Here's how the part is built. I have some questions about the finished solid (model axes, mm). Face numbers are marked on the shaded views. Give positions to 0.01 mm unless a question says otherwise; leave off trailing zeros. Loops run counter-clockwise (first coordinate to the right, second up) from the corner with the lowest first, then second, coordinate; pieces in that order, holes last. Notation, with made-up numbers: (29, 26.25) - (85, 26.25) arc R8 cw to (85, 36.25) - close; hole circle Ø6 at (-26, -29). An arc over 180 degrees is marked (long way). One line per item, written item: value. Start each with the question number.
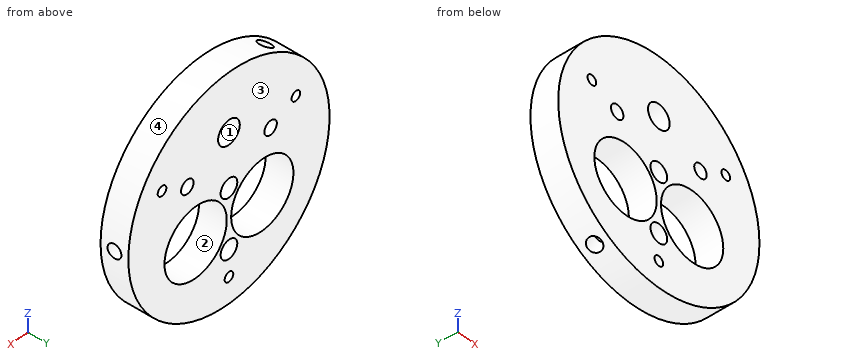
```python
from build123d import *

# Parameters (mm, degrees)
SKETCH1_R               = 38.354
BOSS_EXTRUDE1_DEPTH     = 9.525
SKETCH2_R               = 1.651
SKETCH2_R_2             = 4.1275
SKETCH2_R_3             = 11.8745
SKETCH2_R_4             = 3.175
CUT_EXTRUDE1_DEPTH      = 10.525
SKETCH4_R               = 2.3749
CUT_EXTRUDE2_DEPTH      = 6.35
CIRPATTERN1_COUNT       = 3
SKETCH5_R               = 2.38125
CUT_EXTRUDE3_DEPTH      = 1.0000001
CUT_EXTRUDE3_DEPTH_BACK = 10.5250001


with BuildPart() as part:
    # Sketch1 → Boss-Extrude1 (new body)
    with BuildSketch(Plane(origin=(0, 0, 0), x_dir=(1, 0, 0), z_dir=(0, 1, 0))):
        Circle(SKETCH1_R)
    extrude(amount=BOSS_EXTRUDE1_DEPTH)

    # Sketch2 → Cut-Extrude1 (cut, through all)
    with BuildSketch(Plane(origin=(0, 9.525, 0), x_dir=(1, 0, 0), z_dir=(0, 1, 0))):
        with Locations((0, 29.464)):
            Circle(SKETCH2_R)
        with Locations((25.516572497, -14.732)):
            Circle(SKETCH2_R)
        with Locations((-25.516572497, -14.732)):
            Circle(SKETCH2_R)
        with Locations((0, -18.415)):
            Circle(SKETCH2_R_2)
        with Locations((-12.7, 10.16)):
            Circle(SKETCH2_R_3)
        with Locations((12.7, 10.16)):
            Circle(SKETCH2_R_3)
        with Locations((0, 20.32)):
            Circle(SKETCH2_R_4)
        Circle(SKETCH2_R_4)
    extrude(amount=-CUT_EXTRUDE1_DEPTH, mode=Mode.SUBTRACT)

    # Sketch4 → Cut-Extrude2 (cut)
    with BuildSketch(Plane(origin=(-19.177, 0, -33.215538337), x_dir=(0, -1, 0), z_dir=(-0.5, 0, -0.866025404))):
        with Locations((-4.7625, 0)):
            Circle(SKETCH4_R)
    cut_extrude2 = extrude(amount=-CUT_EXTRUDE2_DEPTH, mode=Mode.SUBTRACT)

    # CirPattern1: Cut-Extrude2 ×3 about axis
    cirpattern1_axis = Axis((0, 0, 0), (0, 1, 0))
    for i in range(1, CIRPATTERN1_COUNT):
        add(cut_extrude2.rotate(cirpattern1_axis, i * 360 / CIRPATTERN1_COUNT), mode=Mode.SUBTRACT)

    # Sketch5 → Cut-Extrude3 (cut, two sides)
    with BuildSketch(Plane(origin=(0, 9.525, 0), x_dir=(1, 0, 0), z_dir=(0, 1, 0))) as cut_extrude3_sk:
        with Locations((-15.875, -10.16)):
            Circle(SKETCH5_R)
        with Locations((15.875, -10.16)):
            Circle(SKETCH5_R)
    extrude(amount=CUT_EXTRUDE3_DEPTH, mode=Mode.SUBTRACT)
    extrude(cut_extrude3_sk.sketch, amount=-CUT_EXTRUDE3_DEPTH_BACK, mode=Mode.SUBTRACT)


solid = part.part
```
(1) If we section it at D-D on z = 11.5: List the corners of the cut face in (x, y) for me (3 decimals).
(2) If we section it at B-B on x = -8: List the corners of the cut face in (y, z) for me (3 decimals), plus the area to 3 significant figures.
(3) If we section it at C-C on y = 4.5: Give the number of separate pieces and of enclosed holes in the cut face, plus the area to 3 significant figures.
(4) If we mould it in two halves opening along X, with no side actions, what happens to the marked faces 1, 2, 3 and 4? For each: pulls with the +X half, pulls with the -X half, needs draft (parallel to the pull), parting line crosses it, or undercut.
(5) Will these pins go through, and if not, where does the flat tip stop? pin 1 (10 mm diameter, centred on x = 0, z = 0, fed in from +Y) (3 decimals); pin 2 (3 mm diameter, centred on x = -1.5, y = 5, fed in from -Z); pin 3 (4 mm diameter, centred on y = 4.76, z = 0, fed in from +X); pin 4 (3 mm diameter, centred on y = 5.5, z = -28.5, fed in from +X).
(6) If we section it at A-A on z = -16: List the corners of the cut face in (x, y) for me (3 decimals), plus the area to 3 significant figures.
(7) Please list where these lines run through material, in increasing order: probe 1 along Z at (x, y) = (0, 4.75) (1 decimal); probe 2 along Z at (x, y) = (-16.5, 9.25); probe 3 along X at (y, z) = (6.5, 14). Write a range as from..to.
Found:
1. outline: (-36.589, 0) - (-17.843, 0) - (-17.843, 9.525) - (-36.589, 9.525) - close; (-13.907, 0) - (13.907, 0) - (13.907, 9.525) - (-13.907, 9.525) - close; (17.843, 0) - (36.589, 0) - (36.589, 9.525) - (17.843, 9.525) - close
2. outline: (0, -37.51) - (9.525, -37.51) - (9.525, -21.065) - (0, -21.065) - close; (0, 0.745) - (9.525, 0.745) - (9.525, 37.51) - (0, 37.51) - close
2. area: 507 mm^2
3. separate pieces: 1
3. enclosed holes: 10
3. area: 3,470 mm^2
4. face 1: undercut
4. face 2: undercut
4. face 3: needs draft
4. face 4: parting line crosses it
5. pin 1: y = 9.525
5. pin 2: z = -38.35
5. pin 3: x = 32
5. pin 4: x = 27.24
6. outline: (-34.857, 0) - (-23.039, 0) - (-23.039, 9.525) - (-34.857, 9.525) - close; (-2.361, 0) - (2.361, 0) - (2.361, 9.525) - (-2.361, 9.525) - close; (23.039, 0) - (34.857, 0) - (34.857, 9.525) - (23.039, 9.525) - close
6. area: 270 mm^2
7. probe 1: -38.4..-31.1, -27.8..-23.5, -17.1..-3.2, 3.2..14.3, 22.5..38.4
7. probe 2: -34.62..-21.41, 1.09..7.86, 12.46..34.62
7. probe 3: -35.71..-27, -24.04..24.04, 27..35.71
